Design review of the part built by this model. Coordinates are the model's own, in mm. Give positions to 0.01 mm unless a question says otherwise; leave off trailing zeros. Loops run counter-clockwise (first coordinate to the right, second up) from the corner with the lowest first, then second, coordinate; pieces in that order, holes last.
Autodesk Inventor part; units mm, degrees
ref_plane "mss_ir_XY" through (0, 0, 0) normal (1, 0, 0) x (0, 0, -1)
ref_plane "mss_ir_YZ" through (0, 0, 0) normal (0, 0, -1) x (0, 1, 0)
ref_plane "mss_ir_ZX" through (0, 0, 0) normal (0, 1, 0) x (1, 0, 0)
sketch "Sketch_2" plane through (0, 0, 0) normal (0, 0, 1) x (1, 0, 0)
  line L0 (5, 0) -> (0, 0)
  arc A0 (0, 3.15) -> (0.15, 3) centre (0.15, 3.15) ccw
  line L1 (0.15, 3) -> (4.85, 3)
  arc A1 (4.85, 3) -> (5, 3.15) centre (4.85, 3.15) ccw
  line L2 (5, 3.15) -> (5, 4.12)
  line L3 (5, 4.12) -> (3.3224, 4.12)
  arc A2 (1.6776, 4.12) -> (3.3224, 4.12) centre (2.5, 4.75) ccw
  line L4 (1.6776, 4.12) -> (0, 4.12)
  line L5 (0, 4.12) -> (0, 3.15)
revolve "Revolution1" add sketch "Sketch_2" angle 360 about axis through (5, 0, 0) along (1, 0, 0)
ref_plane "mss_ir_XY" through (0, 0, 0) normal (1, 0, 0) x (0, 0, -1)
ref_plane "mss_ir_YZ" through (0, 0, 0) normal (0, 0, -1) x (0, 1, 0)
ref_plane "mss_ir_ZX" through (0, 0, 0) normal (0, 1, 0) x (1, 0, 0)
properties part number "W686ZZ Inner ring"
Q1. Wall thickness on line 1 (Z direction, x = 1.6, y = 0); line 2 (Z direction, x = 4.2, y = -0.75); line 3 (Y direction, x = 1.6, z = -1.75): over which ranges is each line inside the solid? List them lowest first.
Results:
line 1: z = -4.12 to -3, 3 to 4.12
line 2: z = -4.05 to -2.9, 2.9 to 4.05
line 3: y = -3.73 to -2.44, 2.44 to 3.73
Q2. Draft analysis for pull direction Y (two halves, no side actions). For faces 1 (the face through (4.149, -3.269, 2.507)), 2 (the face through (3, -3, 0)), state which applies: pulls with the +Y half, pulls with the -Y half, needs draft (parallel to the pull), parting line crosses it, or undercut.
Results:
face 1: parting line crosses it
face 2: undercut
Q3. Take a section at A-A (y = 0). Give the boundary of the cut face in (x, z).
Results:
outline: (0, -4.12) - (1.68, -4.12) arc R1.04 cw to (3.32, -4.12) - (5, -4.12) - (5, -3.15) arc R0.15 ccw to (4.85, -3) - (0.15, -3) arc R0.15 ccw to (0, -3.15) - close; (0, 3.15) arc R0.15 ccw to (0.15, 3) - (4.85, 3) arc R0.15 ccw to (5, 3.15) - (5, 4.12) - (3.32, 4.12) arc R1.04 cw to (1.68, 4.12) - (0, 4.12) - close
Q4. Take a section at C-C (x = 4.35). Give the boundary of the cut face in (y, z), plus the area to 3 significant figures.
Results:
outline: circle Ø8.24 at (0, 0); hole circle Ø6 at (0, 0)
area: 25.1 mm2
Q5. Take a section at D-D (x = 2.3). Give the boundary of the cut face in (y, z), plus the area to 3 significant figures.
Results:
outline: circle Ø7.47 at (0, 0); hole circle Ø6 at (0, 0)
area: 15.5 mm2
Q6. Insertion check: pin 1 (3 mm diameter, centred on x = 1, y = 3, fed in from +Z); pin 2 (2 mm diameter, centred on x = 2.5, z = 3, fed in from -Y); pin 3 (2 mm diameter, centred on x = 1.5, z = -2, fed in from +Y). Each pin has a flat end and moves straight along its axis. Give the tip position at first contact, or say it passes through.
Results:
pin 1: stops at z = 3.84
pin 2: stops at y = -3.33
pin 3: stops at y = 4
